from build123d import *

# Parameters (mm, degrees)
BOSS_EXTRUDE1_DEPTH = 100
SKETCH5_R           = 12.44300021
SKETCH5_W           = 62.427684028
SKETCH5_H           = 20.04871256
CUT_EXTRUDE1_DEPTH  = 100
SKETCH6_W           = 60.250527476
SKETCH6_H           = 14.81598125
CUT_EXTRUDE2_DEPTH  = 100


with BuildPart() as part:
    # Sketch2 → Boss-Extrude1 (new body)
    with BuildSketch(Plane(origin=(0, 0, 0), x_dir=(0, 0, -1), z_dir=(1, 0, 0))):
        Polygon((0, 0), (0, -60), (-60, -60), (-60, -39.746873043), (-19.935380451, -39.746873043), (-19.198069057, 0), align=None)
    extrude(amount=BOSS_EXTRUDE1_DEPTH)

    # Sketch5 → Cut-Extrude1 (cut)
    with BuildSketch(Plane(origin=(0, 0.356005009, 19.191465102), x_dir=(1, 0, 0), z_dir=(0, 0.018546982770064533, 0.99982798992133))):
        with Locations(Location((50, -20.232921797, 0), (0, 0, 270))):
            Circle(SKETCH5_R)
        with Locations((27.151963887, -76.870783424)):
            Rectangle(SKETCH5_W, SKETCH5_H)
    extrude(amount=-CUT_EXTRUDE1_DEPTH, mode=Mode.SUBTRACT)

    # Sketch6 → Cut-Extrude2 (cut)
    with BuildSketch(Plane(origin=(0, -39.746873043, 0), x_dir=(1, 0, 0), z_dir=(0, 1, 0))):
        with Locations((49.391031419, -52.592009375)):
            Rectangle(SKETCH6_W, SKETCH6_H)
    extrude(amount=-CUT_EXTRUDE2_DEPTH, mode=Mode.SUBTRACT)


solid = part.part
Check sheet for the modelled part. Datum: model origin and axes. Units: mm. A direction names the side the tool comes from. Coordinates: 2 decimals unless noted, no trailing zeros. Loops run counter-clockwise (first coordinate to the right, second up) from the corner with the lowest first, then second, coordinate; pieces in that order, holes last. Notation, with made-up numbers: (-15.75, 79.5) -> (32.25, 79.5) arc R29 cw to (32.25, 117.5) -> close; hole circle Ø4 at (-31, 18). An arc over 180 degrees is marked (long way). Answer in a Markdown table with one row per item.
1. Sectioned sample at A-A, the plane z = 51.5. Record the boundary of the cut face in (x, y).
Check values:
| item | result |
|---|---|
| outline | (0, -60) -> (19.27, -60) -> (19.27, -39.75) -> (0, -39.75) -> close; (79.52, -60) -> (100, -60) -> (100, -39.75) -> (79.52, -39.75) -> close |
2. Access from +Z, -Z, +X, -X, +Y, -Y to the whole of each face (thin tool, end or side, straight path). Record for faces 5 (the face through (49, -39.747, 36)), 6 (the face through (19.266, -50, 53)), 7 (the face through (9, -50, 60)).
Check values:
| item | result |
|---|---|
| face 5 | +Z, +X, -X, +Y |
| face 6 | +Z, +Y, -Y |
| face 7 | +Z, +X, -X, +Y, -Y |
3. Sectioned sample at B-B, the plane x = 54. Record the boundary of the cut face in (y, z), then the cut area to 3 significant figures.
Check values:
| item | result |
|---|---|
| outline | (-60, 0) -> (-32.02, 0) -> (-31.65, 19.79) -> (-39.75, 19.94) -> (-39.75, 45.18) -> (-60, 45.18) -> close; (-8.45, 0) -> (0, 0) -> (0, 19.2) -> (-8.09, 19.35) -> close |
| area | 1,230 mm2 |
4. Go/stop test with flat-tipped pins: pin 1 (2 mm diameter, centred on x = 62, z = 36.5, fed in from +Y); pin 2 (22.5 mm diameter, centred on x = 45, y = -52, fed in from +Z). Record where each tip stops, or that it passes through.
Check values:
| item | result |
|---|---|
| pin 1 | stops at y = -39.75 |
| pin 2 | stops at z = 45.18 |
5. Sectioned sample at D-D, the plane x = 31. Record the boundary of the cut face in (y, z).
Check values:
| item | result |
|---|---|
| outline | (-60, 0) -> (0, 0) -> (0, 19.2) -> (-39.75, 19.94) -> (-39.75, 45.18) -> (-60, 45.18) -> close |
6. Material ranges on line 1 along X through (y, z) = (-40, 51); line 2 along Y through (x, z) = (95, 39.5); line 3 along X through (y, z) = (-18, 3), recorded low to high. Write a range as [from, to].
Check values:
| item | result |
|---|---|
| line 1 | x = [0, 19.27], [79.52, 100] |
| line 2 | y = [-60, -39.75] |
| line 3 | x = [0, 37.75], [62.25, 100] |
7. Release check for a two-part mould opening along X. For faces 1 (the face through (79.516, -50, 53)), 2 (the face through (49, -60, 30)), 3 (the face through (37.853, -17.358, 9.757)), 4 (the face through (100, -43, 23)) record: released by +X, released by -X, zero draft, split by the parting line, or undercut.
Check values:
| item | result |
|---|---|
| face 1 | undercut |
| face 2 | zero draft |
| face 3 | undercut |
| face 4 | released by +X |
8. Sectioned sample at C-C, the plane y = -55. Record the boundary of the cut face in (x, z).
Check values:
| item | result |
|---|---|
| outline | (0, 0) -> (100, 0) -> (100, 60) -> (79.52, 60) -> (79.52, 45.18) -> (19.27, 45.18) -> (19.27, 60) -> (0, 60) -> close |
